Solid Edge part; units mm, degrees
sketch "Sketch1" plane through (0, 0, 0) normal (0, 0, 1) x (1, 0, 0)
  arc A0 (-6.8525, 37.382) -> (-1.8525, 42.382) centre (-1.8525, 37.382) cw
  line L0 (-1.8525, 42.382) -> (26.7314, 42.382)
  arc A1 (26.7314, 42.382) -> (31.7314, 37.382) centre (26.7314, 37.382) cw
  line L1 (31.7314, 37.382) -> (31.7314, 34.309)
  arc A2 (31.7314, 34.309) -> (29.7434, 27.3935) centre (18.7097, 34.309) cw
  line L2 (29.7434, 27.3935) -> (26.9077, 22.8691)
  arc A3 (26.9077, 22.8691) -> (30.2548, 17.9831) centre (29.644, 21.1541) ccw
  line L3 (30.2548, 17.9831) -> (42.3551, 20.3139)
  line L4 (42.3551, 20.3139) -> (52.609, 17.5355)
  arc A4 (52.609, 17.5355) -> (58.5185, 5.7573) centre (50.2974, 9.0041) cw
  line L5 (58.5185, 5.7573) -> (51.162, -12.8695)
  arc A5 (51.162, -12.8695) -> (43.8308, -16.3025) centre (45.6786, -10.7039) cw
  line L6 (43.8308, -16.3025) -> (37.7171, -14.2847)
  arc A6 (37.7171, -14.2847) -> (32.7758, -17.5867) centre (36.5355, -17.8647) ccw
  line L7 (32.7758, -17.5867) -> (32.6292, -19.5705)
  arc A7 (32.6292, -19.5705) -> (25.2819, -26.3946) centre (25.2819, -19.0273) cw
  line L8 (25.2819, -26.3946) -> (-11.457, -26.3946)
  arc A8 (-11.457, -26.3946) -> (-23.0909, -14.7608) centre (-11.457, -14.7608) cw
  line L9 (-23.0909, -14.7608) -> (-23.0909, 2.7102)
  arc A9 (-23.0909, 2.7102) -> (-20.4146, 6.5177) centre (-19.0444, 2.7102) cw
  line L10 (-20.4146, 6.5177) -> (-2.4086, 12.9973)
  arc A10 (-2.4086, 12.9973) -> (-0.84, 19.3976) centre (-3.7474, 16.7178) ccw
  line L11 (-0.84, 19.3976) -> (-3.9517, 22.7738)
  arc A11 (-3.9517, 22.7738) -> (-6.8525, 30.201) centre (4.1066, 30.201) cw
  line L12 (-6.8525, 30.201) -> (-6.8525, 37.382)
  circle A12 centre (7.308, -17.457) radius 1.7
  arc A13 (18.0497, -8.2752) -> (14.0663, -8.2752) centre (16.058, -8.457) cw
  arc A14 (14.0663, -8.2752) -> (18.0497, -8.2752) centre (16.058, 2.543) cw
  circle A15 centre (24.1899, 35.9928) radius 1.7
  circle A16 centre (0.2453, 35.9928) radius 1.7
  line L13 (27.2537, -19.157) -> (22.3605, -19.157)
  line L14 (27.2537, -15.757) -> (27.2537, -19.157)
  line L15 (22.3605, -15.757) -> (27.2537, -15.757)
  line L16 (22.3605, -19.157) -> (22.3605, -15.757)
  circle A17 centre (-18.3568, 1.7403) radius 1.7
  circle A18 centre (-12.1594, -21.3884) radius 1.7
  circle A19 centre (47.5876, -11.2739) radius 1.7
  circle A20 centre (51.7456, 12.307) radius 1.7
extrude "Protrusion1" add sketch "Sketch1" against normal blind 4
sketch "Sketch2" plane through (18.0228, 7.9937, -4) normal (0, 0, -1) x (-1, 0, 0)
  circle A0 centre (5.8331, 16.9942) radius 8.6444
  circle A1 centre (24.0074, -14.4162) radius 8.6815
  circle A2 centre (-20.8849, -6.6472) radius 8.9643
extrude "Cutout1" cut sketch "Sketch2" against normal up to next
Verification items for the finished model (mm, model axes). A direction names the side the tool comes from. Give positions to 0.01 mm unless a question says otherwise; leave off trailing zeros. Write each loop counter-clockwise with the first axis right and the second up, starting at its lowest first coordinate (ties: lowest second). Pieces come first, ordered by that corner, then holes. Notation, with made-up numbers: M -16,44.25 L 28,44.25 A10 cw 28,53.25 Z; hole C 26.5,63.25 d3. An arc over 180 degrees is marked long. Use CSV: the item, a comma, the result in double quotes.
1) Cross-section at B-B (y = 9). Enter the section's corners in (x, z), plus the area to 3 significant figures.
Final values:
outline,"M -13.52,-4 L 7.15,-4 L 7.15,0 L -13.52,0 Z; M 24.96,-4 L 34.24,-4 L 34.24,0 L 24.96,0 Z; M 43.57,-4 L 59.14,-4 L 59.14,0 L 43.57,0 Z"
area,"182 mm²"
2) Release check for a two-part mould opening along Y. For faces 1 (the face through (12, 42.382, -2)), 2 (the face through (16.514, 13.534, -1.972)), 3 (the face through (7, -26.395, -2)) record: released by +Y, released by -Y, zero draft, split by the parting line, or undercut.
Final values:
face 1,"released by +Y"
face 2,"undercut"
face 3,"released by -Y"
3) Access from +Z, -Z, +X, -X, +Y, -Y to the whole of each face (thin tool, end or side, straight path). Record for faces 4 (the face through (-22.33, 5.07, -1.97)), 5 (the face through (-2.37, 21.06, -1.97)), 6 (the face through (25, -19.157, -2)), 7 (the face through (28, 8, 0)), 8 (the face through (40.82, -15.31, -1.97)).
Final values:
face 4,"+Z, -Z, -X, +Y"
face 5,"+Z, -Z, -X"
face 6,"+Z, -Z"
face 7,"+Z, +X, -X, +Y, -Y"
face 8,"+Z, -Z, -Y"
4) Cross-section at D-D (y = 28.5). Enter the section's corners in (x, z).
Final values:
outline,"M -6.72,-4 L 4.29,-4 L 4.29,0 L -6.72,0 Z; M 20.09,-4 L 30.36,-4 L 30.36,0 L 20.09,0 Z"
5) Cross-section at A-A (x = -8.5). Enter the section's corners in (y, z).
Final values:
outline,"M -26.39,-4 L -14.73,-4 L -14.73,0 L -26.39,0 Z; M 1.89,-4 L 10.81,-4 L 10.81,0 L 1.89,0 Z"
6) Cross-section at C-C (x = 12.5). Enter the section's corners in (y, z), plus the area to 3 significant figures.
Final values:
outline,"M -26.39,-4 L -7.87,-4 L -7.87,0 L -26.39,0 Z; M 12.95,-4 L 16.35,-4 L 16.35,0 L 12.95,0 Z; M 33.63,-4 L 42.38,-4 L 42.38,0 L 33.63,0 Z"
area,"123 mm²"
7) Go/stop test with flat-tipped pins: pin 1 Ø4.5 at (x, y) = (51.75, 12.31) entering from +Z; pin 2 Ø20 at (x, y) = (16.058, 2.543) entering from +Z; pin 3 Ø2 at (x, z) = (-9.5, -0.5) entering from +Y; pin 4 Ø2 at (y, z) = (35, -1) entering from -X. Record where each tip stops, or that it passes through.
Final values:
pin 1,"z = 0"
pin 2,"through"
pin 3,"y = 10.81"
pin 4,"x = -6.85"
8) Material ranges on line 1 along Y through (x, z) = (23, -2.3); line 2 along Y through (x, z) = (-12.5, -1.3); line 3 along X through (y, z) = (-6, -1.05), recorded low to high.
Final values:
line 1,"-26.39 to -19.16, -15.76 to -5.99, 11.08 to 34.78, 37.21 to 42.38"
line 2,"-26.35 to -23.05, -19.72 to -12.16, -0.69 to 9.37"
line 3,"-23.09 to -14.66, 2.69 to 9.13, 22.99 to 33.77, 44.04 to 53.88"
